from build123d import *

# Parameters (mm, degrees)
SKETCH_1_R          = 6
EXTRUDE_1_DEPTH     = 185
SKETCH_2_R          = 4
EXTRUDE_2_DEPTH     = 20
SKETCH_3_R          = 9.732435518
SKETCH_3_R_2        = 4
CUT_EXTRUDE_1_DEPTH = 10
CUT_EXTRUDE_2_DEPTH = 10


with BuildPart() as part:
    # Эскиз1 → Бобышка-Вытянуть1 (new body)
    with BuildSketch(Plane(origin=(0, 0, 0), x_dir=(1, 0, 0), z_dir=(0, 1, 0))):
        with Locations(Location((0, 0, 0), (0, 0, 270))):
            Circle(SKETCH_1_R)
    extrude(amount=EXTRUDE_1_DEPTH)

    # Эскиз2 → Бобышка-Вытянуть2 (add)
    with BuildSketch(Plane(origin=(0, 185, 0), x_dir=(1, 0, 0), z_dir=(0, 1, 0))):
        with Locations(Location((0, 0, 0), (0, 0, 270))):
            Circle(SKETCH_2_R)
    extrude(amount=EXTRUDE_2_DEPTH)

    # Эскиз3 → Вырез-Вытянуть1 (cut)
    with BuildSketch(Plane.XZ):
        Circle(SKETCH_3_R)
        with Locations(Location((0, 0, 0), (0, 0, 90))):
            Circle(SKETCH_3_R_2, mode=Mode.SUBTRACT)
    extrude(amount=-CUT_EXTRUDE_1_DEPTH, mode=Mode.SUBTRACT)

    # Эскиз4 → Вырез-Вытянуть2 (cut)
    with BuildSketch(Plane.XZ):
        Polygon((-4.486362363, 2.5), (4.2655411, 2.5), (0, 5.300115958), align=None)
    extrude(amount=-CUT_EXTRUDE_2_DEPTH, mode=Mode.SUBTRACT)


solid = part.part
Could you check a few things on this model? Use its own coordinates, in mm. A direction names the side the tool comes from. Give positions to 0.01 mm unless a question says otherwise; leave off trailing zeros. Order: outer loops, then holes, each group sorted by start corner. A loop starts at its lowest first (then second) coordinate and runs counter-clockwise, first axis right, second up. Notation, with made-up numbers: (75.25, 19.5) - (117.25, 19.5) arc R17 cw to (117.25, 23.5) - close; hole circle Ø11 at (14, 39). An arc over 180 degrees is marked (long way). One line per question, with ' | ' between items. Start each with the question number.
Item 1: I need wall thicknesses on probe 1 along Y at (x, z) = (-2.5, 3.75); probe 2 along X at (y, z) = (29, -0.25); probe 3 along X at (y, z) = (23.5, 4.5). Which ranges of each line are inside material? Lowest first, please. Write a range as [from, to].
Item 2: I'm going to push flat-ended pins straight in: pin 1 Ø7 at (x, y) = (-0.5, 4) entering from +Z; pin 2 Ø1.5 at (x, z) = (0.5, -4) entering from -Y; pin 3 Ø2 at (y, z) = (79, 2) entering from -X; pin 4 Ø5 at (x, y) = (-4.5, 61) entering from +Z. Where does each tip first touch, or does it pass through?
Item 3: For faces 1 (the flat face through (0, 5, 2.5)), 2 (the cylindrical face through (0, 5, -4)), 3 (the cylindrical face through (-3.905, 194.86, -0.867)), which set-ups out of +Z, -Z, +X, -X, +Y, -Y let a thin tool reach every point of the face, with its end or its side?
Item 4: I want a section at C-C on y = 22.5. Write out the boundary of the cut face in (x, z).
Item 5: I want a section at B-B on z = 0. Write out the boundary of the cut face in (x, y), then the cut area to 3 significant figures.
Item 6: I want a section at A-A on x = 0. Write out the boundary of the cut face in (y, z), then the cut area to 4 significant figures.
Verdict:
1) probe 1: [10, 185] | probe 2: [-5.99, 5.99] | probe 3: [-3.97, 3.97]
2) pin 1: z = 2.5 | pin 2: y = 0 | pin 3: x = -5.92 | pin 4: z = 5.66
3) face 1: +Z, +X, -X, -Y | face 2: -Y | face 3: +Y
4) outline: circle Ø12 at (0, 0)
5) outline: (-6, 10) - (-4, 10) - (-4, 0) - (4, 0) - (4, 10) - (6, 10) - (6, 185) - (4, 185) - (4, 205) - (-4, 205) - (-4, 185) - (-6, 185) - close | area: 2,340 mm^2
6) outline: (0, -4) - (10, -4) - (10, -6) - (185, -6) - (185, -4) - (205, -4) - (205, 4) - (185, 4) - (185, 6) - (10, 6) - (10, 2.5) - (0, 2.5) - close | area: 2,325 mm^2
